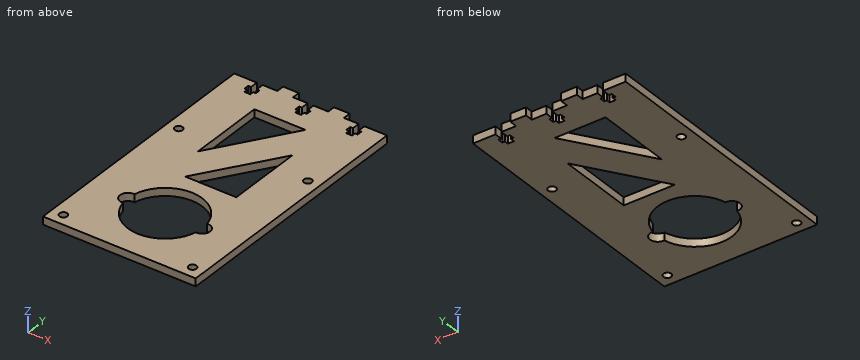
from build123d import *

# Parameters (mm, degrees)
EXTRUDE_1_DEPTH     = 4
SKETCH_3_R          = 2
CUT_EXTRUDE_1_DEPTH = 10
CUT_EXTRUDE_2_DEPTH = 10


with BuildPart() as part:
    # 草图1 → 凸台-拉伸1 (new body)
    with BuildSketch(Plane.XY):
        Polygon((1.5, 0), (1.5, -4), (2.9, -4), (2.9, -6.6), (1.5, -6.6), (1.5, -8.6), (-1.5, -8.6), (-1.5, -6.6), (-2.9, -6.6), (-2.9, -4), (-1.5, -4), (-1.5, 0), (-9, 0), (-9, 4), (-17, 4), (-17, 0), (-24.5, 0), (-24.5, -4), (-23.1, -4), (-23.1, -6.6), (-24.5, -6.6), (-24.5, -8.6), (-27.5, -8.6), (-27.5, -6.6), (-28.9, -6.6), (-28.9, -4), (-27.5, -4), (-27.5, 0), (-39, 0), (-39, -132.712721559), (39, -132.712721559), (39, 0), (27.5, 0), (27.5, -4), (28.9, -4), (28.9, -6.6), (27.5, -6.6), (27.5, -8.6), (24.5, -8.6), (24.5, -6.6), (23.1, -6.6), (23.1, -4), (24.5, -4), (24.5, 0), (17, 0), (17, 4), (9, 4), (9, 0), align=None)
        with BuildLine():
            ThreePointArc((18.578947368, -97.022222394), (0, -82), (-18.578947368, -97.022222394))
            ThreePointArc((-18.578947368, -97.022222394), (-23, -101), (-18.578947368, -104.977777606))
            ThreePointArc((-18.578947368, -104.977777606), (0, -120), (18.578947368, -104.977777606))
            ThreePointArc((18.578947368, -104.977777606), (23, -101), (18.578947368, -97.022222394))
        make_face(mode=Mode.SUBTRACT)
    extrude(amount=EXTRUDE_1_DEPTH)

    # 草图3 → 切除-拉伸1 (cut)
    with BuildSketch(Plane(origin=(0, 0, 0), x_dir=(-1, 0, 0), z_dir=(0, 0, -1))):
        with Locations((33, -126.712721559)):
            Circle(SKETCH_3_R)
        with Locations((33, -46.712721559)):
            Circle(SKETCH_3_R)
        with Locations((-33, -46.712721559)):
            Circle(SKETCH_3_R)
        with Locations((-33, -126.712721559)):
            Circle(SKETCH_3_R)
    extrude(amount=-CUT_EXTRUDE_1_DEPTH, mode=Mode.SUBTRACT)

    # 草图4 → 切除-拉伸2 (cut)
    with BuildSketch(Plane(origin=(0, 0, 0), x_dir=(-1, 0, 0), z_dir=(0, 0, -1))):
        Polygon((16.5, -16.6), (16.5, -55.607703077), (-9.540564725, -16.6), align=None)
        Polygon((9.540564725, -74), (-16.5, -34.992296923), (-16.5, -74), align=None)
    extrude(amount=-CUT_EXTRUDE_2_DEPTH, mode=Mode.SUBTRACT)


solid = part.part
Build history of the part. All positions in model axes, mm. Give positions to 0.01 mm unless a question says otherwise; leave off trailing zeros. Order: outer loops, then holes, each group sorted by start corner. A loop starts at its lowest first (then second) coordinate and runs counter-clockwise, first axis right, second up. Notation, with made-up numbers: M 86,48 L 130,48 A30 ccw 130,70 Z; hole C 49.5,-17.5 d1. An arc over 180 degrees is marked long. Put each result on its own line as item: value.
Item 1: Slice it at B-B, the plane y = -101. Write the cut outline in (x, z).
From the geometry:
outline: M -39,0 L -23,0 L -23,4 L -39,4 Z; M 23,0 L 39,0 L 39,4 L 23,4 Z
Item 2: Probe line 1 (X direction, y = -127, z = 0.3); line 2 (Y direction, x = -33, z = 0.8); line 3 (Y direction, x = -19, z = 3.15). List the from-to ranges inside material, lowest first. Write a range as [from, to].
From the geometry:
line 1: x = [-39, -34.98], [-31.02, 31.02], [34.98, 39]
line 2: y = [-132.71, -128.71], [-124.71, -48.71], [-44.71, 0]
line 3: y = [-132.71, -105], [-97, 0]
Item 3: Flat gauge pins, fed straight in: pin 1 Ø1.2 at (y, z) = (2.5, 1.5) entering from +X; pin 2 Ø1.5 at (x, z) = (-20, 3) entering from +Y; pin 3 Ø2 at (y, z) = (2.5, 1.5) entering from -X. Where does each tip first touch, or does it go through?
From the geometry:
pin 1: stops at x = 17
pin 2: stops at y = 0
pin 3: stops at x = -17
Item 4: Slice it at C-C, the plane x = 4.5. Write the cut outline in (y, z).
From the geometry:
outline: M -132.71,0 L -119.46,0 L -119.46,4 L -132.71,4 Z; M -82.54,0 L -74,0 L -74,4 L -82.54,4 Z; M -52.97,0 L -24.15,0 L -24.15,4 L -52.97,4 Z; M -16.6,0 L 0,0 L 0,4 L -16.6,4 Z
Item 5: Slice it at D-D, the plane x = 21.5. Write the cut outline in (y, z), plus the area to 3 significant figures.
From the geometry:
outline: M -132.71,0 L -104.12,0 L -104.12,4 L -132.71,4 Z; M -97.88,0 L 0,0 L 0,4 L -97.88,4 Z
area: 506 mm2
Item 6: Slice it at A-A, the plane x = 33. Write the cut outline in (y, z).
From the geometry:
outline: M -132.71,0 L -128.71,0 L -128.71,4 L -132.71,4 Z; M -124.71,0 L -48.71,0 L -48.71,4 L -124.71,4 Z; M -44.71,0 L 0,0 L 0,4 L -44.71,4 Z
